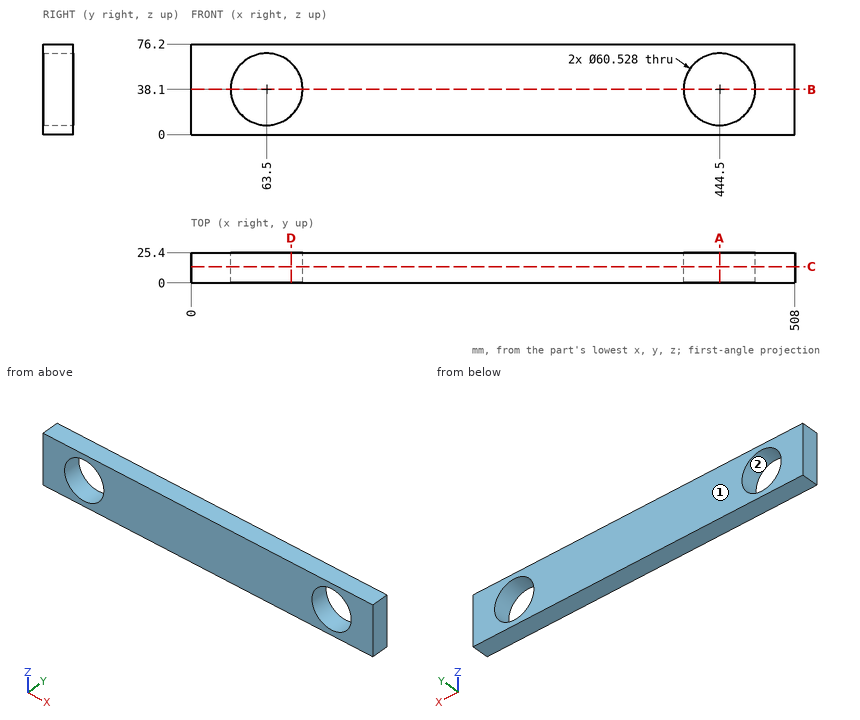
Geometry check sheet. Reference: drawing and pictorial views, mm from the part's lowest x, y, z. Round coordinates to 2 decimals unless told otherwise and drop trailing zeros. Order: outer loops, then holes, each group sorted by start corner. A loop starts at its lowest first (then second) coordinate and runs counter-clockwise, first axis right, second up. Notation, with made-up numbers: M -3.5,-21 L 16.5,-21 A25 ccw 16.5,4 Z; hole C -3.75,-37 d11. An arc over 180 degrees is marked long. One line per item, written item: value. Start each with the question number.
1. Gauge pin test, flat end, axial feed: P1, Ø2, axis at y = 21.5, z = 22, coming from the -X side. Record the tip position at first contact, or that the pin passes through.
2. Section check B-B on z = 38.1. Enter the section's corners in (x, y), and give its area (3 significant figures).
3. Scan lines: line 1 along X through (y, z) = (18.75, 36); line 2 along Z through (x, y) = (444.5, 6.75); line 3 along X through (y, z) = (13, 42). Record each from-to range of solid material in increasing order.
4. Section check C-C on y = 13.5. Enter the section's corners in (x, z), and give its area (3 significant figures).
5. Release check for a two-part mould opening along X. For the marked faces 1 and 2 record: released by +X, released by -X, zero draft, split by the parting line, or undercut.
6. Section check A-A on x = 444.5. Enter the section's corners in (y, z).
7. Section check D-D on x = 84. Enter the section's corners in (y, z).
Results found:
1. P1: x = 0
2. outline: M 0,0 L 33.24,0 L 33.24,25.4 L 0,25.4 Z; M 93.76,0 L 414.24,0 L 414.24,25.4 L 93.76,25.4 Z; M 474.76,0 L 508,0 L 508,25.4 L 474.76,25.4 Z
2. area: 9,830 mm^2
3. line 1: 0 to 33.31, 93.69 to 414.31, 474.69 to 508
3. line 2: 0 to 7.84, 68.36 to 76.2
3. line 3: 0 to 33.49, 93.51 to 414.49, 474.51 to 508
4. outline: M 0,0 L 508,0 L 508,76.2 L 0,76.2 Z; hole C 63.5,38.1 d60.53; hole C 444.5,38.1 d60.53
4. area: 33,000 mm^2
5. face 1: zero draft
5. face 2: undercut
6. outline: M 0,0 L 25.4,0 L 25.4,7.84 L 0,7.84 Z; M 0,68.36 L 25.4,68.36 L 25.4,76.2 L 0,76.2 Z
7. outline: M 0,0 L 25.4,0 L 25.4,15.84 L 0,15.84 Z; M 0,60.36 L 25.4,60.36 L 25.4,76.2 L 0,76.2 Z
